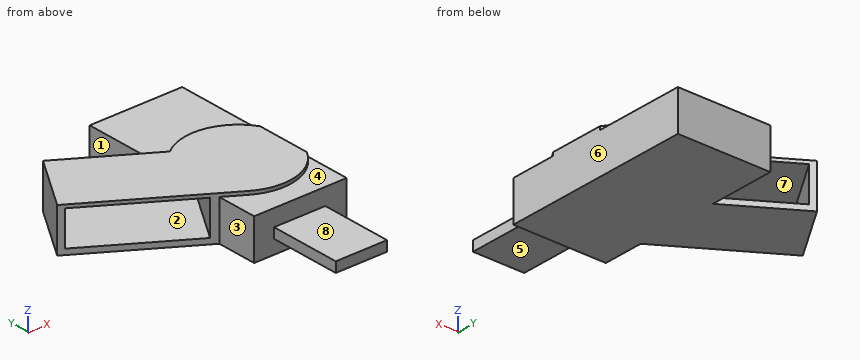
from build123d import *

# Parameters (mm, degrees)
F0_W     = 28.0035007745
F0_H     = 57.5627535582
F1_DEPTH = 12.192
F2_W     = 15.5119162519
F2_H     = 3.0358484946
F3_DEPTH = 21.59
F5_DEPTH = 1.016
F7_DEPTH = 13.208
F8_W     = 33.6042
F8_H     = 10.5041724799
F9_DEPTH = 22.098


with BuildPart() as f1:
    # F0 (on Top) → F1 (new body)
    with BuildSketch(Plane.XY):
        with Locations((-3.8893753663, 12.4460011721)):
            Rectangle(F0_W, F0_H)
    extrude(amount=F1_DEPTH)

    # F2 (on face) → F3 (join)
    with BuildSketch(Plane.XZ.offset(16.335375607)):
        with Locations((-4.1097527137, 5.6689756457)):
            Rectangle(F2_W, F2_H)
    extrude(amount=F3_DEPTH)

    # F4 (on face) → F5 (join)
    with BuildSketch(Plane.XY.offset(12.192)):
        with BuildLine():
            Line((10.112375021, -2.4543297905), (10.112375021, 13.9135444033))
            ThreePointArc((10.112375021, 13.9135444033), (-4.210298008, 21.68161298), (-17.8911257535, 12.8319347765))
            Line((-17.8911257535, 12.8319347765), (-17.8911257535, -1.3727201637))
            ThreePointArc((-17.8911257535, -1.3727201637), (-4.210298008, -10.2223983672), (10.112375021, -2.4543297905))
        make_face()
    extrude(amount=F5_DEPTH)

    # F6 (on face) → F7 (join)
    with BuildSketch(Plane.XY.offset(13.208)):
        with BuildLine():
            ThreePointArc((-17.8911257535, 12.8319347765), (-15.9572228314, 15.8291586852), (-13.4060875251, 18.3221569444))
            Line((-13.4060875251, 18.3221569444), (-38.3101751119, 33.9651258488))
            Line((-38.3101751119, 33.9651258488), (-49.6973358095, 15.8364158124))
            Line((-49.6973358095, 15.8364158124), (-12.0854080322, -7.7887105691))
            ThreePointArc((-12.0854080322, -7.7887105691), (-15.431258916, -4.9815711153), (-17.8911257535, -1.3727201637))
            Line((-17.8911257535, -1.3727201637), (-17.8911257535, 12.8319347765))
        make_face()
    extrude(amount=-F7_DEPTH)

    # F8 (on face) → F9 (cut)
    with BuildSketch(Plane(origin=(-6.9273860037, -11.028611566, 0), x_dir=(0.8468054721, -0.5319027096, 0), z_dir=(-0.5319027096, -0.8468054721, 0))):
        with Locations((-31.8871685294, 6.93991376)):
            Rectangle(F8_W, F8_H)
    extrude(amount=-F9_DEPTH, mode=Mode.SUBTRACT)


solid = f1.part
CAD build for the part. Positions are in the model's coordinates, mm. Face numbers are marked on the shaded views. A direction names the side the tool comes from. Round coordinates to 2 decimals unless told otherwise and drop trailing zeros. Order: outer loops, then holes, each group sorted by start corner. A loop starts at its lowest first (then second) coordinate and runs counter-clockwise, first axis right, second up. Notation, with made-up numbers: M 61,83 L 85,83 A30 ccw 85,115 Z; hole C -31,44 d8. An arc over 180 degrees is marked long. Use one line per item in the form item = value.
Q1. Which spindle directions (+Z, -Z, +X, -X, +Y, -Y) get a long thin tool onto all of the face, cutting with end or side? Do the marked faces 5, 6, 7 and 8. Say none if no direction does.
Recorded:
face_5 = -Z, +X, -X, -Y
face_6 = +Z, -Z, +X, +Y, -Y
face_7 = none
face_8 = +Z, +X, -X, -Y
Q2. Flat gauge pins, fed straight in: P1, Ø4.5, axis at x = -4.5, y = -30, coming from the -Z side; P2, Ø7, axis at x = 2, y = -12.5, coming from the +Z side; P3, Ø2.5, axis at y = -22, z = 5.5, coming from the -X side; P4, Ø13.5, axis at x = 1.5, y = 29, coming from the +Z side. Where does each tip first touch, or does it go through?
Recorded:
P1 = 4.15
P2 = 13.21
P3 = -11.87
P4 = 12.19
Q3. Probe L1, parallel to X at y = -22, z = 5; L2, parallel to X at y = -11.5, z = 7.25; L3, parallel to Y at x = -14.5, z = 12. List the from-to ranges inside material, lowest first.
Recorded:
L1 = -11.87 to 3.65
L2 = -17.89 to 10.11
L3 = -16.34 to 5.28, 19.82 to 41.23
Q4. Saw through at B-B on x = -33.5. Give the cut face in (y, z), then the cut area to 3 significant figures.
Recorded:
outline = M 5.66,0 L 30.94,0 L 30.94,1.69 L 5.66,1.69 Z; M 5.66,12.19 L 30.94,12.19 L 30.94,13.21 L 5.66,13.21 Z
area = 68.4 mm^2
Q5. Saw through at C-C on y = 11.5. Give the cut face in (x, z).
Recorded:
outline = M -42.79,0 L 10.11,0 L 10.11,13.21 L -42.79,13.21 L -42.79,12.19 L -10.59,12.19 L -10.59,1.69 L -42.79,1.69 Z
Q6. Saw through at A-A on z = 6.25. Give the cut face in (x, y).
Recorded:
outline = M -49.7,15.84 L -48.16,14.87 L -36.77,33 L -38.31,33.97 Z; M -19.7,-3 L -17.89,-4.14 L -17.89,-16.34 L -11.87,-16.34 L -11.87,-37.93 L 3.65,-37.93 L 3.65,-16.34 L 10.11,-16.34 L 10.11,41.23 L -17.89,41.23 L -17.89,21.95 L -7.95,15.71 Z
Q7. Two-plate mould, pull along X, no slides. Class the marked faces 1, 2, 3 and 4: +X half, -X half, draft (parallel to the pull), parting line (faces both ways), or undercut.
Recorded:
face_1 = undercut
face_2 = undercut
face_3 = -X half
face_4 = draft
Q8. Saw through at D-D on x = -15.5. Give the cut face in (y, z), then the cut area to 3 significant figures.
Recorded:
outline = M -16.34,0 L 41.23,0 L 41.23,12.19 L 20.45,12.19 L 20.45,1.69 L 3.68,1.69 L 3.68,12.19 L 19.64,12.19 L 19.64,13.21 L -5.64,13.21 L -5.64,12.19 L -16.34,12.19 Z
area = 551 mm^2
